The figure shows three views and two pictorial views of one solid part (mm, origin at its lowest corner). Answer the questions. A direction names the side the tool comes from. Give positions to 0.01 mm unless a question says otherwise; leave off trailing zeros. Loops run counter-clockwise (first coordinate to the right, second up) from the corner with the lowest first, then second, coordinate; pieces in that order, holes last. Notation, with made-up numbers: (66.5, 37) - (101.5, 37) arc R10 ccw to (101.5, 49) - close; hole circle Ø2 at (39.5, -23.5). An arc over 180 degrees is marked (long way). Use a Markdown table: item, result. Add a question column.
Item 1: A cutting plane is placed at B-B (z = 6.75). Determine the outline of the cut face in (x, y) (1 decimal), plus the area to 3 significant figures.
Item 2: Which of the six approach directions +Z, -Z, +X, -X, +Y, -Y give full straight-line access (tool end or side, diameter ignored) to the marked faces 1 and 2?
Item 3: Each of these flat-tipped pins is pushed along its axis until it touches: P1, Ø5, axis at x = 9, y = 6, coming from the +Z side; P2, Ø2, axis at x = 13.5, y = 5, coming from the -Z side. Where does it stop, or does it pass through?
Item 4: A cutting plane is placed at A-A (y = 2). Determine the outline of the cut face in (x, z), plus the area to 3 significant figures.
Item 5: Consider probe 1 along Y at (x, z) = (3.5, 5.25); probe 2 along X at (y, z) = (8.5, 2.5); probe 3 along Z at (x, y) = (17.5, 7.25) (1 decimal). Determine where each line is inside the solid, lowest interval first. Write a range as [from, to].
Item 6: A cutting plane is placed at D-D (z = 1). Determine the outline of the cut face in (x, y), plus the area to 3 significant figures.
Item 7: A cutting plane is placed at C-C (x = 15.75). Determine the outline of the cut face in (y, z).
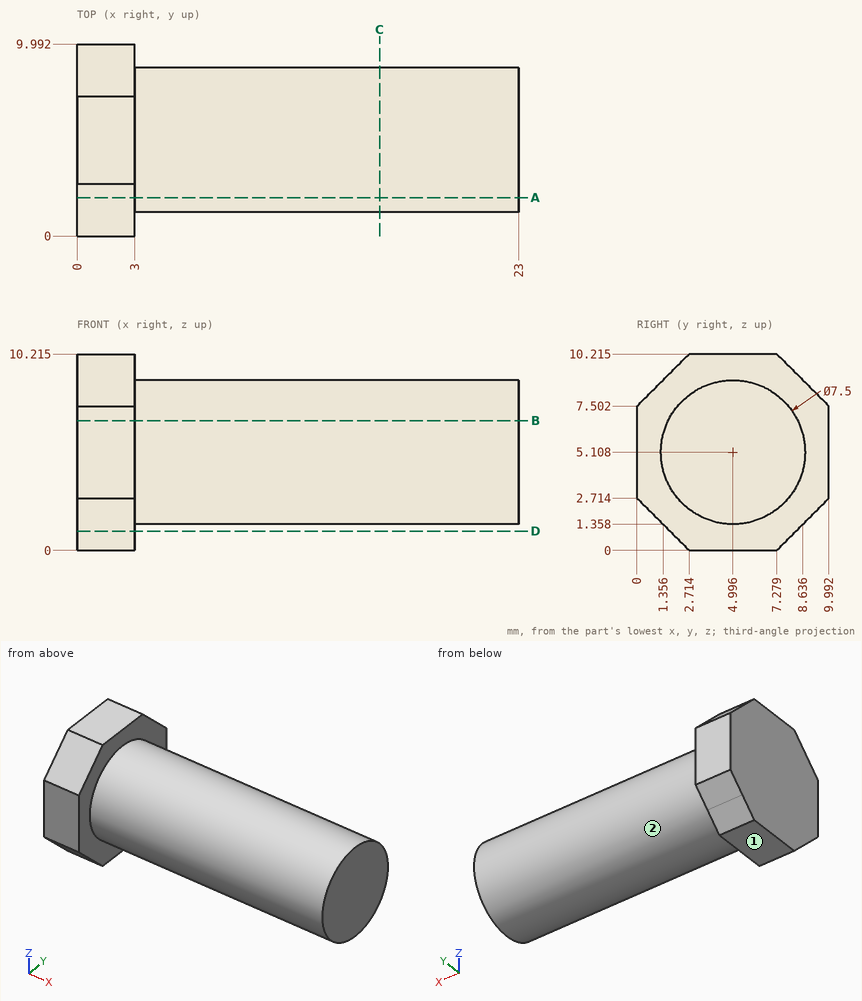
Geometry says:
| question | item | result |
|---|---|---|
| 1 | outline | (0, 0) - (3, 0) - (3, 1.6) - (23, 1.6) - (23, 8.4) - (3, 8.4) - (3, 10) - (0, 10) - close |
| 1 | area | 165 mm² |
| 2 | face 1 | -Z, +X, -X, +Y, -Y |
| 2 | face 2 | +X |
| 3 | P1 | z = 8.86 |
| 3 | P2 | z = 1.36 |
| 4 | outline | (0, 0.71) - (3, 0.71) - (3, 2.85) - (23, 2.85) - (23, 7.36) - (3, 7.36) - (3, 9.5) - (0, 9.5) - close |
| 4 | area | 117 mm² |
| 5 | probe 1 | [1.25, 8.74] |
| 5 | probe 2 | [0, 3] |
| 5 | probe 3 | [2.1, 8.1] |
| 6 | outline | (0, 1.71) - (3, 1.71) - (3, 8.28) - (0, 8.28) - close |
| 6 | area | 19.7 mm² |
| 7 | outline | circle Ø7.5 at (5, 5.11) |
